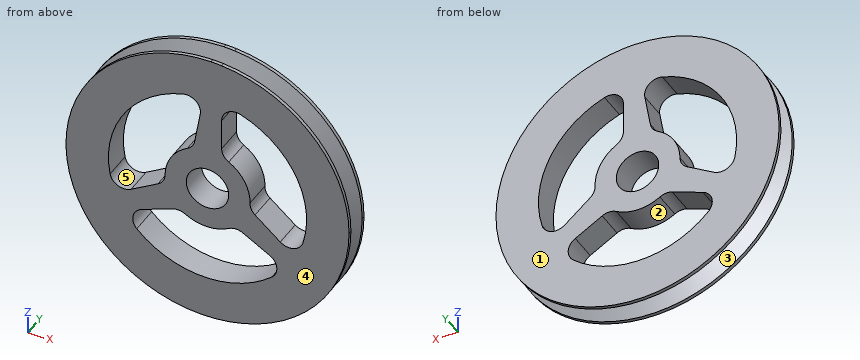
```python
from build123d import *

# Parameters (mm, degrees)
F0_R     = 1.5
F1_DEPTH = 1


# Not quite as in the source:
# - ends of sketch curves that miss each other by under 0.0002 mm in the source are joined


with BuildPart() as f1:
    # F0 (on Front) → F1 (new body, symmetric)
    with BuildSketch(Plane.XZ):
        with BuildLine():
            ThreePointArc((0.2401150839, 9.9971168217), (-7.1554577365, -6.985658493), (10, 0))
            ThreePointArc((10, 0), (7.4161984871, 6.7082039325), (1, 9.9498743711))
            ThreePointArc((1, 9.9498743711), (0.6205086012, 9.9807298869), (0.2401150839, 9.9971168217))
        make_face()
        with BuildLine():
            ThreePointArc((4.5488093998, -5.3205575877), (-0.3054811817, -6.9933311982), (-4.9954209636, -4.90364858))
            ThreePointArc((-4.9954209636, -4.90364858), (-5.2574280938, -3.9837438223), (-4.6268502112, -3.2645470249))
            Line((-4.6268502112, -3.2645470249), (-2.4485091499, -2.4636990679))
            ThreePointArc((-2.4485091499, -2.4636990679), (-2.0029061262, -2.4073466036), (-1.5775862521, -2.551709548))
            ThreePointArc((-1.5775862521, -2.551709548), (-0.0451926266, -2.9996595851), (1.5, -2.5980762114))
            ThreePointArc((1.5, -2.5980762114), (2, -2.4641016151), (2.5, -2.5980762114))
            Line((2.5, -2.5980762114), (4.3989794856, -3.6944525285))
            ThreePointArc((4.3989794856, -3.6944525285), (4.8947614013, -4.4687262228), (4.5488093998, -5.3205575877))
        make_face(mode=Mode.SUBTRACT)
        with BuildLine():
            ThreePointArc((-0.9093714051, 3.3523206591), (-1.0833702513, 2.9382408884), (-1.4210521656, 2.6420845449))
            ThreePointArc((-1.4210521656, 2.6420845449), (-2.5751850901, 1.5389677552), (-3, 0))
            ThreePointArc((-3, 0), (-3.1339745962, -0.5), (-3.5, -0.8660254038))
            Line((-3.5, -0.8660254038), (-5.3989794856, -1.962401721))
            ThreePointArc((-5.3989794856, -1.962401721), (-6.3174111322, -2.0046246076), (-6.8821427332, -1.2791057034))
            ThreePointArc((-6.8821427332, -1.2791057034), (-5.9036618838, 3.7612200629), (-1.7489737597, 6.7779857471))
            ThreePointArc((-1.7489737597, 6.7779857471), (-0.8213093054, 6.5449381989), (-0.5137555498, 5.6392433348))
            Line((-0.5137555498, 5.6392433348), (-0.9093714051, 3.3523206591))
        make_face(mode=Mode.SUBTRACT)
        Circle(F0_R, mode=Mode.SUBTRACT)
        with BuildLine():
            Line((1, 3.4641016151), (1, 5.6568542495))
            ThreePointArc((1, 5.6568542495), (1.4226497308, 6.4733508304), (2.3333333333, 6.5996632911))
            ThreePointArc((2.3333333333, 6.5996632911), (6.2091430656, 3.2321111353), (6.7443947233, -1.8743371671))
            ThreePointArc((6.7443947233, -1.8743371671), (6.0787373992, -2.5611943766), (5.140605761, -2.3746963099))
            Line((5.140605761, -2.3746963099), (3.357880555, -0.8886215913))
            ThreePointArc((3.357880555, -0.8886215913), (3.0862763775, -0.5308942848), (2.9986384177, -0.090374997))
            ThreePointArc((2.9986384177, -0.090374997), (2.6203777167, 1.4606918299), (1.5, 2.5980762114))
            ThreePointArc((1.5, 2.5980762114), (1.1339745962, 2.9641016151), (1, 3.4641016151))
        make_face(mode=Mode.SUBTRACT)
    extrude(amount=F1_DEPTH, both=True)

    # F2 (on Right) → F3 (revolve, cut)
    with BuildSketch(Plane.YZ):
        Polygon((-0.75, 10), (0, 8.5), (0, 10), align=None)
        Polygon((0, 10), (0, 8.5), (0.75, 10), align=None)
    revolve(axis=Axis((0, 4.7748805955, 0), (0, 1, 0)), mode=Mode.SUBTRACT)


solid = f1.part
```
Input: part model. Units: mm. Frame: model coordinates. Face numbers are marked on the shaded views. A direction names the side the tool comes from. Give positions to 0.01 mm unless a question says otherwise; leave off trailing zeros. Loops run counter-clockwise (first coordinate to the right, second up) from the corner with the lowest first, then second, coordinate; pieces in that order, holes last.
1) Reachability of the marked faces 3, 4 and 5 from +Z, -Z, +X, -X, +Y, -Y: full face, straight path, thin tool, end or side. Return the list, or none.
A:
face 3: none
face 4: +Z, -Z, +X, -X, -Y
face 5: +Y, -Y
2) Section query B-B on z = 0.75. Count the separate pieces of the cut face and the enclosed holes in it, and give its area (3 significant figures).
A:
separate pieces: 4
enclosed holes: 0
area: 16.2 mm2
3) Line query: L1, parallel to Z at x = 2, y = -0.9; L2, parallel to Z at x = 0.25, y = -0.3; L3, parallel to Y at x = 8.25, z = -5.5. Output: solid intervals per line, ascending.
A:
L1: z = -9.8 to -6.71, -2.46 to 2.24, 6.66 to 9.8
L2: z = -9.1 to -7, -2.99 to -1.48, 1.48 to 9.1
L3: y = -1 to -0.71, 0.71 to 1
4) Contact query for a flat-ended pin moving along its axis: pin 1 (1 mm diameter, centred on y = 0.5, z = 5, fed in from +X). Output: stop coordinate, or through.
A:
pin 1: stops at x = 8.9
5) Section query A-A on y = 0.25. Return the cut outline in (x, z).
A:
outline: circle Ø18 at (0, 0); hole (-6.88, -1.28) arc R1 ccw to (-5.4, -1.96) - (-3.5, -0.87) arc R1 ccw to (-3, 0) arc R3 cw to (-1.42, 2.64) arc R1 ccw to (-0.91, 3.35) - (-0.51, 5.64) arc R1 ccw to (-1.75, 6.78) arc R7 ccw to start; hole (-5, -4.9) arc R7 ccw to (4.55, -5.32) arc R1 ccw to (4.4, -3.69) - (2.5, -2.6) arc R1 ccw to (1.5, -2.6) arc R3 cw to (-1.58, -2.55) arc R1 ccw to (-2.45, -2.46) - (-4.63, -3.26) arc R1 ccw to start; hole circle Ø3 at (0, 0); hole (1, 3.46) arc R1 ccw to (1.5, 2.6) arc R3 cw to (3, -0.09) arc R1 ccw to (3.36, -0.89) - (5.14, -2.37) arc R1 ccw to (6.74, -1.87) arc R7 ccw to (2.33, 6.6) arc R1 ccw to (1, 5.66) - close
6) Mould query, pull axis Z, two halves, no side actions, for the marked faces 1 and 2. Classes: released by +Z, released by -Z, zero draft, split by the parting line, or undercut.
A:
face 1: zero draft
face 2: undercut
